```python
from build123d import *

# Parameters (mm, degrees)
SKETCH_1_W          = 3.4
SKETCH_1_H          = 29.8
SKETCH_1_W_2        = 2
EXTRUDE_1_DEPTH     = 16
CUT_EXTRUDE_START   = 1
SKETCH_1_3_W        = 1.4
SKETCH_1_3_H        = 29.8
CUT_EXTRUDE_1_DEPTH = 14
SKETCH_4_W          = 35.141232352
SKETCH_4_H          = 2.32880635
CUT_EXTRUDE_4_DEPTH = 5.8
CHAMFER_2_SIZE      = 1
CHAMFER_1_SIZE      = 0.6
CUT_EXTRUDE_2_REACH = 15.8
SKETCH_2_R          = 1.2
SKETCH_3_R          = 2.05
CUT_EXTRUDE_3_DEPTH = 1


with BuildPart() as part:
    # Sketch 1 → Extrude 1 (new body)
    with BuildSketch(Plane(origin=(0, 0, 0), x_dir=(1, 0, 0), z_dir=(0, 1, 0))):
        with Locations((1.7, 14.9)):
            Rectangle(SKETCH_1_W, SKETCH_1_H)
        Polygon((-10.4, 19.4), (-10.4, 10.4), (0, 0), (0, 29.8), align=None)
        with Locations((2.4, 14.9)):
            Rectangle(SKETCH_1_W_2, SKETCH_1_H)
    extrude(amount=EXTRUDE_1_DEPTH)

    # Sketch 1_3 → Cut-Extrude 1 (cut)
    with BuildSketch(Plane(origin=(0, 0, 0), x_dir=(1, 0, 0), z_dir=(0, 1, 0)).offset(CUT_EXTRUDE_START)):
        Polygon((-10.4, 19.4), (-10.4, 10.4), (0, 0), (0, 29.8), align=None)
        with Locations((0.7, 14.9)):
            Rectangle(SKETCH_1_3_W, SKETCH_1_3_H)
    extrude(amount=CUT_EXTRUDE_1_DEPTH, mode=Mode.SUBTRACT)

    # Sketch 4 → Cut-Extrude 4 (cut)
    with BuildSketch(Plane.ZY.offset(10.4)):
        with Locations((-15.55462397, -0.164403175)):
            Rectangle(SKETCH_4_W, SKETCH_4_H)
    extrude(amount=-CUT_EXTRUDE_4_DEPTH, mode=Mode.SUBTRACT)

    # Chamfer 2
    chamfer_2_edges = [part.edges().sort_by_distance(p)[0] for p in [
        (3.4, 16, -14.9),
        (3.4, 8, -29.8),
        (3.4, 8, 0),
        (3.4, 0, -14.9),
    ]]
    chamfer(chamfer_2_edges, length=CHAMFER_2_SIZE)

    # Chamfer 1
    chamfer_1_edges = [part.edges().sort_by_distance(p)[0] for p in [
        (1.2, 16, -29.8),
        (-5.2, 16, -24.6),
        (-10.4, 16, -14.9),
        (-5.2, 16, -5.2),
        (-2.3, 0, -2.3),
        (-4.6, 0, -14.9),
        (1.2, 16, 0),
        (1.2, 0, 0),
        (-2.3, 0, -27.5),
        (1.2, 0, -29.8),
    ]]
    chamfer(chamfer_1_edges, length=CHAMFER_1_SIZE)

    # Sketch 2 → Cut-Extrude 2 (cut, up to next)
    with BuildSketch(Plane(origin=(3.4, 0, 0), x_dir=(0, 0, -1), z_dir=(1, 0, 0)), mode=Mode.PRIVATE) as cut_extrude_2_sk1:
        with Locations((8.9, 8)):
            Circle(SKETCH_2_R)
    cut_extrude_2_tool1 = extrude(cut_extrude_2_sk1.sketch, amount=-CUT_EXTRUDE_2_REACH, mode=Mode.PRIVATE) & part.part
    add(cut_extrude_2_tool1.solids().sort_by_distance((3.4, 8, -8.9))[0], mode=Mode.SUBTRACT)
    # Sketch 2 → Cut-Extrude 2 (cut, up to next)
    with BuildSketch(Plane(origin=(3.4, 0, 0), x_dir=(0, 0, -1), z_dir=(1, 0, 0)), mode=Mode.PRIVATE) as cut_extrude_2_sk2:
        with Locations((20.9, 8)):
            Circle(SKETCH_2_R)
    cut_extrude_2_tool2 = extrude(cut_extrude_2_sk2.sketch, amount=-CUT_EXTRUDE_2_REACH, mode=Mode.PRIVATE) & part.part
    add(cut_extrude_2_tool2.solids().sort_by_distance((3.4, 8, -20.9))[0], mode=Mode.SUBTRACT)

    # Sketch 3 → Cut-Extrude 3 (cut)
    with BuildSketch(Plane(origin=(3.4, 0, 0), x_dir=(0, 0, -1), z_dir=(1, 0, 0))):
        with Locations((8.9, 8)):
            Circle(SKETCH_3_R)
        with Locations((20.9, 8)):
            Circle(SKETCH_3_R)
    extrude(amount=-CUT_EXTRUDE_3_DEPTH, mode=Mode.SUBTRACT)


solid = part.part
```
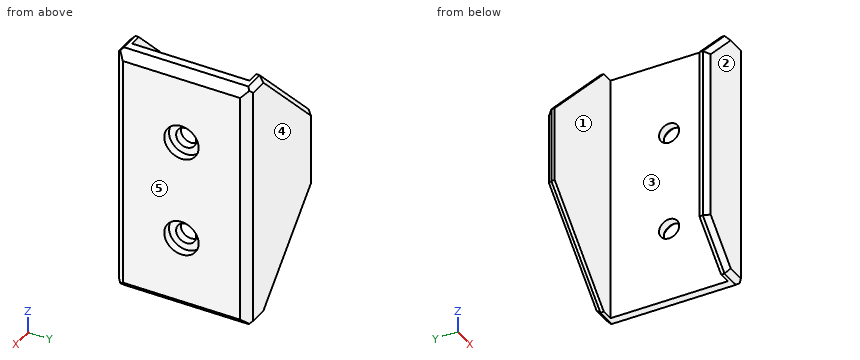
Geometry check sheet. Reference: the model listing, model coordinates, mm. Face numbers are marked on the shaded views. A direction names the side the tool comes from. Give positions to 0.01 mm unless a question says otherwise; leave off trailing zeros. Loops run counter-clockwise (first coordinate to the right, second up) from the corner with the lowest first, then second, coordinate; pieces in that order, holes last. Notation, with made-up numbers: M -18,45.5 L -4,45.5 A13 ccw -4,65.5 Z; hole C 51.5,71.5 d7. An arc over 180 degrees is marked long. Write item = value, one per line. Start each with the question number.
1. Tool access check on the marked faces 1 and 2. Record the directions out of +Z, -Z, +X, -X, +Y, -Y that give a thin tool (end or side, any length) a straight path to the whole face; none if there is none.
2. Section check C-C, the plane z = -20.9. Enter the section's corners in (x, y), plus the area to 3 significant figures.
3. Go/stop test with flat-tipped pins: P1, Ø4.5, axis at y = 8, z = -20.9, coming from the -X side; P2, Ø4, axis at y = 8, z = -20.9, coming from the +X side. Record where each tip stops, or that it passes through.
4. Section check B-B, the plane z = -11.25. Enter the section's corners in (x, y).
5. Section check D-D, the plane y = 13.5. Enter the section's corners in (x, z).
6. Draft check along Y on the marked faces 3, 4 and 5. Enter one of: +Y half, -Y half, draft (parallel to the pull), parting line (faces both ways), or undercut.
7. Section check A-A, the plane y = 8. Enter the section's corners in (x, z).
8. Thickness scan on probe 1 along Y at (x, z) = (2.15, -8.9); probe 2 along Y at (x, z) = (0.75, -23); probe 3 along Z at (x, y) = (2.25, 7.25). Record the ranges inside material, lowest first.
Values follow:
q1.face_1 = +Z, -Z, -X
q1.face_2 = +Z, -Z, +X, -X, -Y
q2.outline = M -8.9,15 L 1.4,15 L 1.4,9.2 L 2.4,9.2 L 2.4,10.05 L 3.4,10.05 L 3.4,15 L 2.4,16 L -8.05,16 L -8.9,15.4 Z; M -4.6,0.6 L -4,0 L 2.4,0 L 3.4,1 L 3.4,5.95 L 2.4,5.95 L 2.4,6.8 L 1.4,6.8 L 1.4,1 L -4.6,1 Z
q2.area = 40.4 mm^2
q3.P1 = 1.4
q3.P2 = 2.4
q4.outline = M -10.4,15 L 1.4,15 L 1.4,1 L -4.6,1 L -4.6,0.6 L -4,0 L 2.4,0 L 3.4,1 L 3.4,15 L 2.4,16 L -9.8,16 L -10.4,15.4 Z
q5.outline = M 1.4,-29.8 L 2.4,-29.8 L 3.4,-28.8 L 3.4,-1 L 2.4,0 L 1.4,0 Z
q6.face_3 = undercut
q6.face_4 = +Y half
q6.face_5 = draft
q7.outline = M 1.4,-29.8 L 2.4,-29.8 L 3.4,-28.8 L 3.4,-22.95 L 2.4,-22.95 L 2.4,-22.1 L 1.4,-22.1 Z; M 1.4,-19.7 L 2.4,-19.7 L 2.4,-18.85 L 3.4,-18.85 L 3.4,-10.95 L 2.4,-10.95 L 2.4,-10.1 L 1.4,-10.1 Z; M 1.4,-7.7 L 2.4,-7.7 L 2.4,-6.85 L 3.4,-6.85 L 3.4,-1 L 2.4,0 L 1.4,0 Z
q8.probe_1 = 0 to 6.8, 9.2 to 16
q8.probe_2 = 0 to 1, 15 to 16
q8.probe_3 = -29.8 to -21.84, -19.96 to -9.84, -7.96 to 0
